Check sheet for the modelled part. Datum: model origin and axes. Units: mm. A direction names the side the tool comes from. Give positions to 0.01 mm unless a question says otherwise; leave off trailing zeros. Order: outer loops, then holes, each group sorted by start corner. A loop starts at its lowest first (then second) coordinate and runs counter-clockwise, first axis right, second up.
Item 1: Sectioned sample at D-D on y = -11. Record the boundary of the cut face in (x, z), and give its area (3 significant figures).
Item 2: Sectioned sample at C-C on z = -16. Record the boundary of the cut face in (x, y), and give its area (3 significant figures).
Item 3: Access from +Z, -Z, +X, -X, +Y, -Y to the whole of each face (thin tool, end or side, straight path). Record for faces 1 (the cylindrical face through (18.544, 0.108, 13.149)), 2 (the flat face through (-32.5, 5, 0)), 3 (the flat face through (0, 18, -19.5)), 4 (the cylindrical face through (-24.892, 17.635, 9.044)), 5 (the flat face through (10.5, -15, 0)).
Item 4: Sectioned sample at A-A on y = 15. Record the boundary of the cut face in (x, z).
Item 5: Release check for a two-part mould opening along Y. For faces 6 (the conical face through (21.374, 0.118, 6.307)), 7 (the flat face through (-31.5, -17, -0.3)), 8 (the cylindrical face through (23.5, 17.64, 9.55)) record: released by +Y, released by -Y, zero draft, split by the parting line, or undercut.
Item 6: Sectioned sample at B-B on x = 15.5. Record the boundary of the cut face in (y, z), and give its area (3 significant figures).
Item 7: Material ranges on line 1 along X through (y, z) = (23.5, 12); line 2 along Y through (x, z) = (-21, 12.25); line 3 along X through (y, z) = (0, 5.5), recorded low to high.
Item 8: Gauge pin test, flat ends, axial feed: P1, Ø5.5, axis at x = 21, y = 0, coming from the +Z side; P2, Ø4, axis at x = -25, z = 11.5, coming from the +Y side; P3, Ø2, axis at x = -6.5, z = 14.5, coming from the -Y side. Record the tip position at first contact, or that the pin passes through.
from build123d import *

# Parameters (mm, degrees)
EXTRUDE_1_DEPTH      = 19.5
EXTRUDE_1_DEPTH_BACK = 19.5


with BuildPart() as part:
    # Sketch 1 → Extrude 1 (new, two sides: drawn at the far end of the back side and taken through both)
    with BuildSketch(Plane.XY.offset(-EXTRUDE_1_DEPTH_BACK)):
        with BuildLine():
            Line((-32.5, 25), (-32.5, -16))
            Line((-32.5, -16), (-30.5, -18))
            Line((-30.5, -18), (-10.5, -18))
            Line((-10.5, -18), (-10.5, -12.727922061))
            ThreePointArc((-10.5, -12.727922061), (0, 16.5), (10.5, -12.727922061))
            Line((10.5, -12.727922061), (10.5, -18))
            Line((10.5, -18), (30.5, -18))
            Line((30.5, -18), (32.5, -16))
            Line((32.5, -16), (32.5, 25))
            Line((32.5, 25), (-32.5, 25))
        make_face()
    extrude(amount=EXTRUDE_1_DEPTH + EXTRUDE_1_DEPTH_BACK)

    # Sketch 2 → Cut-Revolve 1 (revolve, cut)
    with BuildSketch(Plane(origin=(21, 0, 0), x_dir=(0, 0, -1), z_dir=(1, 0, 0)), mode=Mode.PRIVATE) as cut_revolve_1_sk:
        Polygon((-19.5, 0), (-19.5, 3), (-18.9585, 2.4585), (-7.5, 2.4585), (-6.080584363, 0), align=None)
    revolve(cut_revolve_1_sk.sketch.rotate(Axis((21, 0, 6.080584363), (0, 0, 1)), 270), axis=Axis((21, 0, 6.080584363), (0, 0, 1)), mode=Mode.SUBTRACT)

    # Sketch 3 → Cut-Revolve 2 (revolve, cut)
    with BuildSketch(Plane(origin=(-21, 0, 0), x_dir=(0, 0, -1), z_dir=(1, 0, 0)), mode=Mode.PRIVATE) as cut_revolve_2_sk:
        Polygon((-19.5, 0), (-19.5, 3), (-18.9585, 2.4585), (-7.5, 2.4585), (-6.080584363, 0), align=None)
    revolve(cut_revolve_2_sk.sketch.rotate(Axis((-21, 0, 6.080584363), (0, 0, 1)), 270), axis=Axis((-21, 0, 6.080584363), (0, 0, 1)), mode=Mode.SUBTRACT)

    # Sketch 4 → Cut-Revolve 3 (revolve, cut)
    with BuildSketch(Plane(origin=(25, 0, 0), x_dir=(0, 0, -1), z_dir=(1, 0, 0)), mode=Mode.PRIVATE) as cut_revolve_3_sk:
        Polygon((-11.5, 25), (-8.5, 25), (-9.0415, 24.4585), (-9.0415, 11), (-11.5, 9.580584363), align=None)
    revolve(cut_revolve_3_sk.sketch.rotate(Axis((25, 9.580584363, 11.5), (0, 1, 0)), 180), axis=Axis((25, 9.580584363, 11.5), (0, 1, 0)), mode=Mode.SUBTRACT)

    # Sketch 5 → Cut-Revolve 4 (revolve, cut)
    with BuildSketch(Plane(origin=(25, 0, 0), x_dir=(0, 0, -1), z_dir=(1, 0, 0)), mode=Mode.PRIVATE) as cut_revolve_4_sk:
        Polygon((11.5, 25), (14.5, 25), (13.9585, 24.4585), (13.9585, 11), (11.5, 9.580584363), align=None)
    revolve(cut_revolve_4_sk.sketch.rotate(Axis((25, 9.580584363, -11.5), (0, 1, 0)), 180), axis=Axis((25, 9.580584363, -11.5), (0, 1, 0)), mode=Mode.SUBTRACT)

    # Sketch 6 → Cut-Revolve 5 (revolve, cut)
    with BuildSketch(Plane(origin=(-25, 0, 0), x_dir=(0, 0, -1), z_dir=(1, 0, 0)), mode=Mode.PRIVATE) as cut_revolve_5_sk:
        Polygon((-11.5, 25), (-8.5, 25), (-9.0415, 24.4585), (-9.0415, 11), (-11.5, 9.580584363), align=None)
    revolve(cut_revolve_5_sk.sketch.rotate(Axis((-25, 9.580584363, 11.5), (0, 1, 0)), 180), axis=Axis((-25, 9.580584363, 11.5), (0, 1, 0)), mode=Mode.SUBTRACT)

    # Sketch 7 → Cut-Revolve 6 (revolve, cut)
    with BuildSketch(Plane(origin=(-25, 0, 0), x_dir=(0, 0, -1), z_dir=(1, 0, 0)), mode=Mode.PRIVATE) as cut_revolve_6_sk:
        Polygon((11.5, 25), (14.5, 25), (13.9585, 24.4585), (13.9585, 11), (11.5, 9.580584363), align=None)
    revolve(cut_revolve_6_sk.sketch.rotate(Axis((-25, 9.580584363, -11.5), (0, 1, 0)), 180), axis=Axis((-25, 9.580584363, -11.5), (0, 1, 0)), mode=Mode.SUBTRACT)


solid = part.part
Report:
1. outline: (-32.5, -19.5) - (-12.3, -19.5) - (-12.3, 19.5) - (-32.5, 19.5) - close; (12.3, -19.5) - (32.5, -19.5) - (32.5, 19.5) - (12.3, 19.5) - close
1. area: 1,580 mm2
2. outline: (-32.5, -16) - (-30.5, -18) - (-10.5, -18) - (-10.5, -12.73) arc R16.5 cw (long way) to (10.5, -12.73) - (10.5, -18) - (30.5, -18) - (32.5, -16) - (32.5, 25) - (-32.5, 25) - close
2. area: 1,880 mm2
3. face 1: +Z
3. face 2: +Z, -Z, -X, +Y, -Y
3. face 3: -Z, +X, -X, +Y, -Y
3. face 4: +Y
3. face 5: +Z, -Z, -Y
4. outline: (-32.5, -19.5) - (-6.87, -19.5) - (-6.87, 19.5) - (-32.5, 19.5) - close; (6.87, -19.5) - (32.5, -19.5) - (32.5, 19.5) - (6.87, 19.5) - close; hole circle Ø4.92 at (-25, -11.5); hole circle Ø4.92 at (-25, 11.5); hole circle Ø4.92 at (25, -11.5); hole circle Ø4.92 at (25, 11.5)
5. face 6: undercut
5. face 7: released by -Y
5. face 8: zero draft
6. outline: (-18, -19.5) - (-5.66, -19.5) - (-5.66, 19.5) - (-18, 19.5) - close; (5.66, -19.5) - (25, -19.5) - (25, 19.5) - (5.66, 19.5) - close
6. area: 1,240 mm2
7. line 1: x = -32.5 to -27.41, -22.59 to 22.59, 27.41 to 32.5
7. line 2: y = -18 to -2.46, 2.46 to 25
7. line 3: x = -32.5 to -16.5, 16.5 to 32.5
8. P1: stops at z = 19.25
8. P2: stops at y = 10.74
8. P3: stops at y = 14.7
